Check sheet for the modelled part. Datum: model origin and axes. Units: mm. Face numbers are marked on the shaded views. Coordinates: 2 decimals unless noted, no trailing zeros. Write each loop counter-clockwise with the first axis right and the second up, starting at its lowest first coordinate (ties: lowest second). Pieces come first, ordered by that corner, then holes. Notation, with made-up numbers: (36.5, 87.5) -> (62.5, 87.5) arc R18 cw to (62.5, 116.5) -> close; hole circle Ø8 at (67.25, 74.5). An arc over 180 degrees is marked (long way). One line per item, written item: value. Start each with the question number.
1) Sectioned sample at A-A on y = -11.5. Enter the section's corners in (x, z).
2) Sectioned sample at C-C on x = -12. Enter the section's corners in (y, z), plus the area to 3 significant figures.
3) Sectioned sample at B-B on z = -14. Enter the section's corners in (x, y), plus the area to 3 significant figures.
4) Scan lines: line 1 along X through (y, z) = (-24.7, 14); line 2 along Z through (x, y) = (17.5, -18.5); line 3 along X through (y, z) = (-19.25, -16). Record each from-to range of solid material in increasing order. Write a range as [from, to].
5) Draft check along X on the marked faces 1, 2 and 3. Enter one of: +X half, -X half, draft (parallel to the pull), parting line (faces both ways), or undercut.
6) Gauge pin test, flat ends, axial feed: P1, Ø6, axis at x = 24.3, z = -4.95, coming from the -Y side; P2, Ø7.5, axis at y = -20.5, z = 16, coming from the -X side; P3, Ø4, axis at x = -24.3, z = -4.95, coming from the -Y side; P4, Ø1.5, axis at y = 0, z = 4, coming from the +X side. Record the tip position at first contact, or that the pin passes through.
7) Sectioned sample at D-D on z = 9. Enter the section's corners in (x, y).
```python
from build123d import *

# Parameters (mm, degrees)
SKETCH1_W           = 60.5
SKETCH1_H           = 40
SKETCH1_W_2         = 43
SKETCH1_H_2         = 23
BOSS_EXTRUDE1_DEPTH = 2.5
BOSS_EXTRUDE2_DEPTH = 5
BOSS_EXTRUDE3_DEPTH = 5
SKETCH4_R           = 2.25
CUT_EXTRUDE1_DEPTH  = 172.982842356
BOSS_EXTRUDE4_START = -29
SKETCH6_W           = 20
SKETCH6_H           = 5
BOSS_EXTRUDE4_DEPTH = 24
SKETCH7_W           = 14
SKETCH7_H           = 6
CUT_EXTRUDE3_DEPTH  = 177.123713622
FILLET1_R           = 2
FILLET2_R           = 2
FILLET3_R           = 1.5
CUT_EXTRUDE4_REACH  = 166.861
SKETCH8_R           = 2
BOSS_EXTRUDE5_DEPTH = 3
FILLET4_R           = 2


with BuildPart() as part:
    # Sketch1 → Boss-Extrude1 (new, symmetric)
    with BuildSketch(Plane(origin=(0, 0, 0), x_dir=(1, 0, 0), z_dir=(0, 1, 0))):
        Rectangle(SKETCH1_W, SKETCH1_H)
        Rectangle(SKETCH1_W_2, SKETCH1_H_2, mode=Mode.SUBTRACT)
    extrude(amount=BOSS_EXTRUDE1_DEPTH, both=True)

    # Sketch2 → Boss-Extrude2 (add)
    with BuildSketch(Plane(origin=(0, 2.5, 0), x_dir=(1, 0, 0), z_dir=(0, 1, 0))):
        with BuildLine():
            Line((30.25, 20), (30.25, -20))
            ThreePointArc((30.25, -20), (47.256913802, -12.826981202), (58.25, 2))
            ThreePointArc((58.25, 2), (42.044671251, 7.569488613), (30.25, 20))
        make_face()
        with BuildLine():
            Line((35.25, 6.366833624), (35.25, -13.722672005))
            ThreePointArc((35.25, -13.722672005), (44.009484688, -9.018930074), (50.750559549, -1.710601274))
            ThreePointArc((50.750559549, -1.710601274), (42.564834707, 1.49249914), (35.25, 6.366833624))
        make_face(mode=Mode.SUBTRACT)
    extrude(amount=-BOSS_EXTRUDE2_DEPTH)

    # Sketch3 → Boss-Extrude3 (add)
    with BuildSketch(Plane(origin=(0, 2.5, 0), x_dir=(1, 0, 0), z_dir=(0, 1, 0))):
        with BuildLine():
            Line((-30.25, 20), (-30.25, -20))
            Line((-30.25, -20), (30.25, -20))
            ThreePointArc((30.25, -20), (-71.163797142, -21.66706635), (-170.25, 0))
            ThreePointArc((-170.25, 0), (-99.592440555, 5.397083884), (-30.25, 20))
        make_face()
    extrude(amount=-BOSS_EXTRUDE3_DEPTH)

    # Sketch4 → Cut-Extrude1 (cut, through all)
    with BuildSketch(Plane(origin=(0, 2.5, 0), x_dir=(1, 0, 0), z_dir=(0, 1, 0))):
        with Locations(Location((-24.3, 4.95, 0), (0, 0, 270))):
            Circle(SKETCH4_R)
        with Locations(Location((-24.3, -4.95, 0), (0, 0, 270))):
            Circle(SKETCH4_R)
        with Locations(Location((24.3, -4.95, 0), (0, 0, 90))):
            Circle(SKETCH4_R)
        with Locations(Location((24.3, 4.95, 0), (0, 0, 90))):
            Circle(SKETCH4_R)
    extrude(amount=-CUT_EXTRUDE1_DEPTH, mode=Mode.SUBTRACT)

    # Sketch6 → Boss-Extrude4 (add)
    with BuildSketch(Plane(origin=(0, 2.5, 0), x_dir=(1, 0, 0), z_dir=(0, 1, 0)).offset(BOSS_EXTRUDE4_START)):
        with Locations((10.3, 14)):
            Rectangle(SKETCH6_W, SKETCH6_H)
        with Locations((10.3, -14)):
            Rectangle(SKETCH6_W, SKETCH6_H)
    extrude(amount=BOSS_EXTRUDE4_DEPTH)

    # Sketch7 → Cut-Extrude3 (cut, through all)
    with BuildSketch(Plane.XY.offset(16.5)):
        with Locations((10.3, -19.5)):
            Rectangle(SKETCH7_W, SKETCH7_H)
    extrude(amount=-CUT_EXTRUDE3_DEPTH, mode=Mode.SUBTRACT)

    # Fillet1
    fillet1_edges = [part.edges().sort_by_distance(p)[0] for p in [
        (-170.25, 0, 0),
    ]]
    fillet(fillet1_edges, radius=FILLET1_R)

    # Fillet2
    fillet2_edges = [part.edges().sort_by_distance(p)[0] for p in [
        (58.25, 0, -2),
        (30.25, 0, -20),
    ]]
    fillet(fillet2_edges, radius=FILLET2_R)

    # Fillet3
    fillet3_edges = [part.edges().sort_by_distance(p)[0] for p in [
        (35.25, 0, -6.366833624),
        (35.25, 0, 13.722672005),
        (50.750559549, 0, 1.710601274),
    ]]
    fillet(fillet3_edges, radius=FILLET3_R)

    # Sketch8 → Cut-Extrude4 (cut, up to next)
    with BuildSketch(Plane.XZ.offset(26.5), mode=Mode.PRIVATE) as cut_extrude4_sk1:
        with Locations(Location((6.3, 14, 0), (0, 0, 270))):
            Circle(SKETCH8_R)
    cut_extrude4_tool1 = extrude(cut_extrude4_sk1.sketch, amount=-CUT_EXTRUDE4_REACH, mode=Mode.PRIVATE) & part.part
    # Sketch8 → Cut-Extrude4 (cut, up to next)
    with BuildSketch(Plane.XZ.offset(26.5), mode=Mode.PRIVATE) as cut_extrude4_sk2:
        with Locations(Location((14.3, 14, 0), (0, 0, 270))):
            Circle(SKETCH8_R)
    cut_extrude4_tool2 = extrude(cut_extrude4_sk2.sketch, amount=-CUT_EXTRUDE4_REACH, mode=Mode.PRIVATE) & part.part
    cut_extrude4_1 = cut_extrude4_tool1.solids().sort_by_distance((6.3, -26.5, 14))[0]
    add(cut_extrude4_1, mode=Mode.SUBTRACT)
    cut_extrude4_2 = cut_extrude4_tool2.solids().sort_by_distance((14.3, -26.5, 14))[0]
    add(cut_extrude4_2, mode=Mode.SUBTRACT)
    cut_extrude4 = cut_extrude4_1 + cut_extrude4_2  # Cut-Extrude4 as one shape, for the pattern or mirror that repeats it

    # Sketch9 → Boss-Extrude5 (add, symmetric)
    with BuildSketch(Plane(origin=(10.3, 0, 0), x_dir=(0, 0, -1), z_dir=(1, 0, 0))):
        Polygon((-20, -2.5), (-16.5, -16.5), (-16.5, -2.5), align=None)
    boss_extrude5 = extrude(amount=BOSS_EXTRUDE5_DEPTH, both=True)

    # Mirror1: Cut-Extrude4, Boss-Extrude5 across plane
    add(cut_extrude4.mirror(Plane.XY), mode=Mode.SUBTRACT)
    add(boss_extrude5.mirror(Plane.XY))

    # Fillet4
    # the kernel refuses this fillet: 2 mm, written as the material it adds along each edge
    with BuildSketch(Plane(origin=(20.3, -2.5, 16.5), x_dir=(0, 0, 1), z_dir=(-1, 0, 0)), Plane(origin=(0.3, -2.5, -16.5), x_dir=(0, 0, -1), z_dir=(1, 0, 0)), Plane(origin=(8.3, -2.5, -16.5), x_dir=(0, 0, -1), z_dir=(1, 0, 0)), Plane(origin=(12.3, -2.5, 16.5), x_dir=(0, 0, 1), z_dir=(-1, 0, 0))) as fillet4_piece_1:
        with BuildLine():
            CenterArc((FILLET4_R, -FILLET4_R), FILLET4_R, 90, 90)
            Line((0, -FILLET4_R), (0, 0))
            Line((0, 0), (FILLET4_R, 0))
        make_face()
    extrude(amount=12)
    with BuildSketch(Plane(origin=(7.3, -2.5, 11.5), x_dir=(-1, 0, 0), z_dir=(0, 0, 1))) as fillet4_piece_2_section:
        with BuildLine():
            CenterArc((FILLET4_R, FILLET4_R), FILLET4_R, 180, 90)
            Line((0, FILLET4_R), (0, 0))
            Line((0, 0), (FILLET4_R, 0))
        make_face()
    fillet4_piece_2 = extrude(amount=13.5, mode=Mode.PRIVATE)
    fillet4_piece_2 = split(fillet4_piece_2, bisect_by=Plane(origin=(6.847209771, -4.337920215, 19.540519946), z_dir=(0, 0.242535625036333, -0.9701425001453319)), keep=Keep.TOP, mode=Mode.PRIVATE)
    add(fillet4_piece_2)
    with BuildSketch(Plane(origin=(13.3, -2.5, 20), x_dir=(0, 0, 1), z_dir=(-1, 0, 0))) as fillet4_piece_3:
        with BuildLine():
            CenterArc((FILLET4_R * 0.780776406404, -FILLET4_R), FILLET4_R, 90, 75.963756532)
            Line((-FILLET4_R * 0.189366093741, -FILLET4_R * 0.757464374964), (0, 0))
            Line((0, 0), (FILLET4_R * 0.780776406404, 0))
        make_face()
    extrude(amount=6)
    with BuildSketch(Plane(origin=(13.3, -2.5, 11.5), x_dir=(1, 0, 0), z_dir=(0, 0, 1))) as fillet4_piece_4_section:
        with BuildLine():
            CenterArc((FILLET4_R, -FILLET4_R), FILLET4_R, 90, 90)
            Line((0, -FILLET4_R), (0, 0))
            Line((0, 0), (FILLET4_R, 0))
        make_face()
    fillet4_piece_4 = extrude(amount=13.5, mode=Mode.PRIVATE)
    fillet4_piece_4 = split(fillet4_piece_4, bisect_by=Plane(origin=(13.752790229, -4.337920215, 19.540519946), z_dir=(0, 0.242535625036333, -0.9701425001453319)), keep=Keep.TOP, mode=Mode.PRIVATE)
    add(fillet4_piece_4)
    with BuildSketch(Plane(origin=(13.3, -2.5, -11.5), x_dir=(1, 0, 0), z_dir=(0, 0, -1))) as fillet4_piece_5_section:
        with BuildLine():
            CenterArc((FILLET4_R, FILLET4_R), FILLET4_R, 180, 90)
            Line((0, FILLET4_R), (0, 0))
            Line((0, 0), (FILLET4_R, 0))
        make_face()
    fillet4_piece_5 = extrude(amount=8.5, mode=Mode.PRIVATE)
    fillet4_piece_5 = split(fillet4_piece_5, bisect_by=Plane(origin=(13.752790229, -4.337920215, -19.540519946), z_dir=(0, 0.242535625036333, 0.9701425001453319)), keep=Keep.TOP, mode=Mode.PRIVATE)
    add(fillet4_piece_5)
    with BuildSketch(Plane(origin=(7.3, -2.5, -11.5), x_dir=(-1, 0, 0), z_dir=(0, 0, -1))) as fillet4_piece_6_section:
        with BuildLine():
            CenterArc((FILLET4_R, -FILLET4_R), FILLET4_R, 90, 90)
            Line((0, -FILLET4_R), (0, 0))
            Line((0, 0), (FILLET4_R, 0))
        make_face()
    fillet4_piece_6 = extrude(amount=8.5, mode=Mode.PRIVATE)
    fillet4_piece_6 = split(fillet4_piece_6, bisect_by=Plane(origin=(6.847209771, -4.337920215, -19.540519946), z_dir=(0, 0.242535625036333, 0.9701425001453319)), keep=Keep.TOP, mode=Mode.PRIVATE)
    add(fillet4_piece_6)
    with BuildSketch(Plane(origin=(13.3, -2.5, 20), x_dir=(0, 0, 1), z_dir=(-1, 0, 0))) as fillet4_piece_7a_section:
        with BuildLine():
            CenterArc((FILLET4_R * 0.780776406404, -FILLET4_R), FILLET4_R, 90, 75.963756532)
            Line((-FILLET4_R * 0.189366093741, -FILLET4_R * 0.757464374964), (0, 0))
            Line((0, 0), (FILLET4_R * 0.780776406404, 0))
        make_face()
    fillet4_piece_7a = extrude(amount=9.903882032, mode=Mode.PRIVATE)
    fillet4_piece_7a = split(fillet4_piece_7a, bisect_by=Plane(origin=(7.3, -2.834860191, 20.261450936), z_dir=(-1, 0, 0)), keep=Keep.TOP, mode=Mode.PRIVATE)
    with BuildSketch(Plane(origin=(7.3, -2.5, 16.5), x_dir=(-1, 0, 0), z_dir=(0, 0, 1))) as fillet4_piece_7b_section:
        with BuildLine():
            CenterArc((FILLET4_R, FILLET4_R), FILLET4_R, 180, 90)
            Line((0, FILLET4_R), (0, 0))
            Line((0, 0), (FILLET4_R, 0))
        make_face()
    fillet4_piece_7b = extrude(amount=8.5, mode=Mode.PRIVATE)
    fillet4_piece_7b = fillet4_piece_7b & Plane(origin=(-27.619084703, -2.967404811, -414.868675855), x_dir=(0.1319097290212544, 0, 0.9912617330400378), z_dir=(0, 1, 0)) * Cylinder(438.702172555, 25, mode=Mode.PRIVATE)
    fillet4_piece_7b = split(fillet4_piece_7b, bisect_by=Plane(origin=(6.852193926, -2.662257848, 19.959435538), z_dir=(0, -0.242535625036333, 0.9701425001453319)), keep=Keep.TOP, mode=Mode.PRIVATE)
    fillet4_piece_7 = fillet4_piece_7a & fillet4_piece_7b
    add(fillet4_piece_7)
    with BuildSketch(Plane(origin=(13.3, -2.5, 16.5), x_dir=(1, 0, 0), z_dir=(0, 0, 1))) as fillet4_piece_8a_section:
        with BuildLine():
            CenterArc((FILLET4_R, -FILLET4_R), FILLET4_R, 90, 90)
            Line((0, -FILLET4_R), (0, 0))
            Line((0, 0), (FILLET4_R, 0))
        make_face()
    fillet4_piece_8a = extrude(amount=8.5, mode=Mode.PRIVATE)
    fillet4_piece_8a = fillet4_piece_8a & Plane(origin=(-27.619084703, -2.981369523, -414.868675855), x_dir=(0.1319097290212544, 0, 0.9912617330400378), z_dir=(0, 1, 0)) * Cylinder(438.702172555, 25, mode=Mode.PRIVATE)
    fillet4_piece_8a = split(fillet4_piece_8a, bisect_by=Plane(origin=(13.730097047, -2.74600268, 19.93849933), z_dir=(0, -0.242535625036333, 0.9701425001453319)), keep=Keep.TOP, mode=Mode.PRIVATE)
    with BuildSketch(Plane(origin=(17.203882032, -2.5, 20), x_dir=(0, 0, 1), z_dir=(-1, 0, 0))) as fillet4_piece_8b_section:
        with BuildLine():
            CenterArc((FILLET4_R * 0.780776406404, -FILLET4_R), FILLET4_R, 90, 75.963756532)
            Line((-FILLET4_R * 0.189366093741, -FILLET4_R * 0.757464374964), (0, 0))
            Line((0, 0), (FILLET4_R * 0.780776406404, 0))
        make_face()
    fillet4_piece_8b = extrude(amount=9.903882032, mode=Mode.PRIVATE)
    fillet4_piece_8b = fillet4_piece_8b & Plane(origin=(-27.619084703, -2.834877125, -414.868675855), x_dir=(0.1319097290212544, 0, 0.9912617330400378), z_dir=(0, 1, 0)) * Cylinder(438.702172555, 27, mode=Mode.PRIVATE)
    fillet4_piece_8b = split(fillet4_piece_8b, bisect_by=Plane(origin=(13.3, -2.834877125, 20.261389272), z_dir=(1, 0, 0)), keep=Keep.TOP, mode=Mode.PRIVATE)
    fillet4_piece_8 = fillet4_piece_8a & fillet4_piece_8b
    add(fillet4_piece_8)


solid = part.part
```
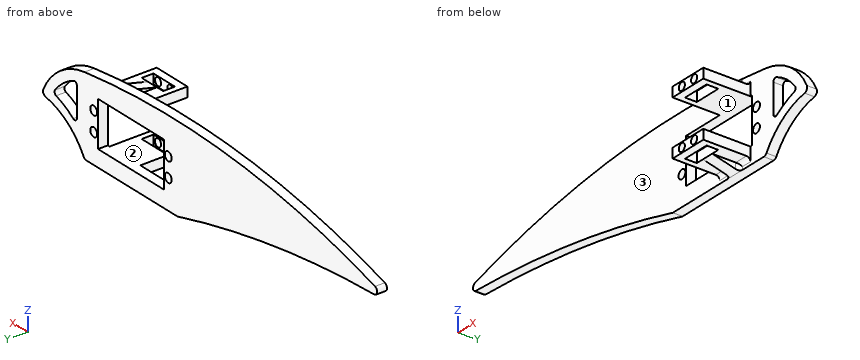
Answers:
1. outline: (0.3, -16.5) -> (7.3, -16.5) -> (7.3, -17.75) -> (13.3, -17.75) -> (13.3, -16.5) -> (20.3, -16.5) -> (20.3, -11.5) -> (0.3, -11.5) -> close; (0.3, 11.5) -> (20.3, 11.5) -> (20.3, 16.5) -> (13.3, 16.5) -> (13.3, 17.75) -> (7.3, 17.75) -> (7.3, 16.5) -> (0.3, 16.5) -> close
2. outline: (-2.5, -20) -> (2.5, -20) -> (2.5, -11.5) -> (-2.5, -11.5) -> close; (-2.5, 11.5) -> (2.5, 11.5) -> (2.5, 23.56) -> (-2.5, 23.56) -> close
2. area: 103 mm2
3. outline: (-53.67, -2.5) -> (0.3, -2.5) -> (0.3, -26.5) -> (4.3, -26.5) -> (4.3, -22.5) -> (3.3, -22.5) -> (3.3, -16.5) -> (17.3, -16.5) -> (17.3, -22.5) -> (16.3, -22.5) -> (16.3, -26.5) -> (20.3, -26.5) -> (20.3, -2.5) -> (34.55, -2.5) -> (34.55, 2.5) -> (-53.67, 2.5) -> close; (8.3, -26.5) -> (12.3, -26.5) -> (12.3, -22.5) -> (8.3, -22.5) -> close
3. area: 805 mm2
4. line 1: x = [0.3, 4.3], [8.3, 12.3], [16.3, 20.3]
4. line 2: z = [-16.5, -11.5], [11.5, 16.5]
4. line 3: x = [0.3, 3.3], [17.3, 20.3]
5. face 1: undercut
5. face 2: undercut
5. face 3: draft
6. P1: stops at y = -2.5
6. P2: stops at x = 0.3
6. P3: passes through
6. P4: stops at x = 55.68
7. outline: (-140.73, -2.5) -> (-21.5, -2.5) -> (-21.5, 2.5) -> (-140.73, 2.5) -> close; (21.5, -2.5) -> (35.25, -2.5) -> (35.25, 2.5) -> (21.5, 2.5) -> close; (44.03, -2.5) -> (51.39, -2.5) -> (51.39, 2.5) -> (44.03, 2.5) -> close
